Can you work these out from the model? Positions are in its coordinate system, mm. Face numbers are marked on the shaded views. A direction names the side the tool comes from. Round coordinates to 2 decimals unless told otherwise and drop trailing zeros. Order: outer loops, then holes, each group sorted by start corner. A loop starts at its lowest first (then second) coordinate and runs counter-clockwise, first axis right, second up. Notation, with made-up numbers: (-6, 37) -> (26, 37) arc R7 ccw to (26, 41) -> close; hole circle Ø5 at (13.5, -7). An arc over 180 degrees is marked (long way). Use a Markdown table: item, result. Add a question column.
Q1. If we section it at A-A on x = -2.15: List the corners of the cut face in (y, z) for me, plus the area to 3 significant figures.
Q2. For the marked faces 1 and 2, which set-ups out of +Z, -Z, +X, -X, +Y, -Y let a thin tool reach every point of the face, with its end or its side?
Q3. If we section it at B-B on x = 9.5: List the corners of the cut face in (y, z) for me.
Q4. I'm going to push flat-ended pins straight in: pin 1 Ø2 at (x, z) = (7.5, 3.5) entering from +Y; pin 2 Ø5 at (x, y) = (26, 4.5) entering from -Z; pin 3 Ø4 at (y, z) = (-2.5, 1) entering from +X; pin 4 Ø4 at (x, y) = (14, -3) entering from -Z. Where does each tip first touch, or does it pass through?
Q5. I need wall thicknesses on line 1 along X through (y, z) = (0, -3.9); line 2 along X through (y, z) = (0, -1.6); line 3 along X through (y, z) = (1.75, 4). Which ranges of each line are inside material? Lowest first, please. Write a range as [from, to].
Autodesk Inventor part; units mm, degrees
ref_plane "Work Plane1" through (16, 0, 0) normal (0, 0, -1) x (1, 0, 0)
ref_plane "YZ Plane" through (0, 0, 0) normal (1, 0, 0) x (0, 1, 0)
ref_plane "XZ Plane" through (0, 0, 0) normal (0, 1, 0) x (-1, 0, 0)
sketch "草图1" plane through (0, 0, 0) normal (0, 0, 1) x (1, 0, 0)
  line L0 (0, 4.45) -> (0, 3)
  line L1 (12, 3) -> (30, 3)
  line L2 (30, 3) -> (30, 0)
  line L3 (30, 0) -> (-0.1501, 0)
  line L4 (-6.1801, 0) -> (36.03, 0)
  line L5 (-0.1501, 0) -> (-0.1501, 4.45)
  line L6 (-0.1501, 4.45) -> (0, 4.45)
  line L7 (12, 3) -> (11.3866, 3)
  line L8 (11.3866, 3) -> (0, 3)
  line L9 (0, -0.89) -> (0, 5.34)
  line L10 (11.3866, 3) -> (11.3866, 0) construction
  line L11 (12, 3) -> (12, 0) construction
  dimension "d0" = 30
  dimension "d1" = 18
  dimension "d2" = 6
  dimension "d9" = 0.1501
  dimension "d10" = 8.9
  dimension "d13" = 0.6135
  dimension "d14" = 6
revolve "轴承体" add sketch "草图1" angle 360 about axis through (30, 0, 0) along (-1, 0, 0)
sketch "草图2" plane through (-0.1501, 0, 0) normal (-1, 0, 0) x (0, 0, 1)
  line L0 (0, 5.7735) -> (5, 2.8868)
  line L1 (5, 2.8868) -> (5, -2.8868)
  line L2 (5, -2.8868) -> (0, -5.7735)
  line L3 (0, -5.7735) -> (-5, -2.8868)
  line L4 (-5, -2.8868) -> (-5, 2.8868)
  line L5 (-5, 2.8868) -> (0, 5.7735)
  point P0 (0, 0)
  point P1 (0, 0)
  dimension "d11" = 10
extrude "头" add sketch "草图2" along normal blind 3.85
sketch "草图3" plane through (0, 0, 0) normal (0, 0, 1) x (1, 0, 0)
  line L0 (-4.0001, 5) -> (-4.0001, 5.7735)
  line L1 (-4.0001, 5.7735) -> (-3.5535, 5.7735)
  line L2 (-3.5535, 5.7735) -> (-4.0001, 5)
  line L3 (-4.7701, 0) -> (0.6199, 0)
  line L4 (-0.1501, 5.7735) -> (-4.0001, 5.7735)
  line L5 (-4.0001, 2.8868) -> (-4.0001, 5.7735)
  dimension "d5" = 30
  dimension "d25" = 10
revolve "倒角1" cut sketch "草图3" angle 360 about axis through (-10, 0, 0) along (1, 0, 0)
sketch "草图4" plane through (0, 0, 0) normal (0, 0, 1) x (1, 0, 0)
  circle A0 centre (-2.15, 0) radius 0.8
  line L0 (-3.54, 0) -> (0.59, 0)
  point P0 (0, 0)
  dimension "d18" = 1.6
  dimension "d19" = 2.15
extrude "孔" cut sketch "草图4" along normal through all both and the other way through all
pattern_circular "IDS_ARRAYHOLE" count 2 over 60 about axis through (-10, 0, 0) along (1, 0, 0) of "孔"
fillet "圆角1" radius 0.25 1 edges at (0, -3, 0)
thread "螺纹"
chamfer "倒角2" distance 0.6135 distance2 0.6136 1 edges at (30, -3, 0) measured on face at (30, -0.5525, 1.8157)
ref_plane "Work Plane1" through (16, 0, 0) normal (0, 0, -1) x (1, 0, 0)
equation "\"d0\" = NLG"
equation "\"d1\" = GEL"
equation "\"d2\" = GD"
equation "\"d10\" = SD2"
equation "\"d13\" = GAL"
equation "\"d14\" = BDM"
equation "\"d11\" = SW"
equation "\"d3\" = KOH - SD"
equation "\"d5\" = ANG1"
equation "\"d25\" = SW0"
equation "\"d18\" = BOR"
equation "\"d24\" = RR"
equation "\"d15\" = GEL"
equation "\"d6\" = -0.5 * SPD + 0.5 * GD"
equation "\"NLG\" = 30"
equation "\"GD\" = NND"
equation "\"BDM\" = NND"
equation "\"KOH\" = 4"
equation "\"GEL\" = 18"
equation "\"SW\" = 10"
equation "\"SW0\" = SW"
equation "\"SPD\" = NND - 1.2269 * PTC"
equation "\"SD2\" = SDH"
equation "\"SD\" = WFT"
equation "\"ANG1\" = 30deg"
equation "\"GAL\" = 0.61345 * PTC"
equation "\"GUL\" = 0.61345 * PTC"
equation "\"DIST\" = 2"
equation "\"BOR\" = 1.6"
equation "\"RR\" = 0.25"
equation "\"WFT\" = 0.15"
equation "\"FAWI\" = 45deg"
equation "\"PTC\" = 1"
equation "\"THREADDIA\" = 6"
equation "\"E0\" = 1.155 * SW"
equation "\"TOA\" = 30deg"
equation "\"NND\" = 6"
equation "\"GD1\" = THREADDIA - 1.2269 * PTC"
equation "\"SDH\" = 8.9"
properties part number "螺栓 GB 32.1 M6 x 30" material "钢，软"
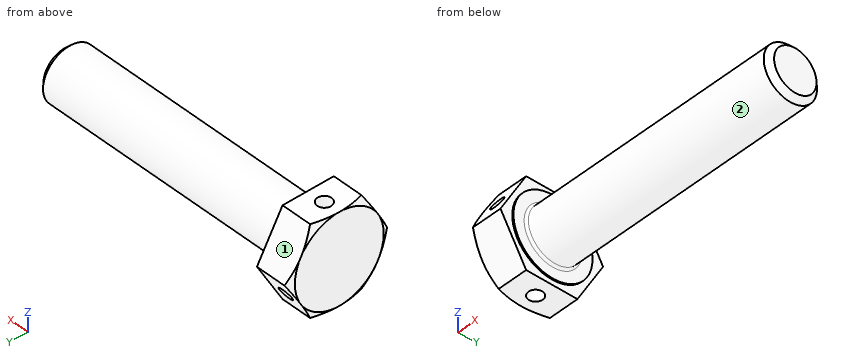
Answer below:
| question | item | result |
|---|---|---|
| 1 | outline | (-5.77, 0) -> (-2.89, -5) -> (-0.8, -5) -> (-0.8, -0.46) -> (-4.73, 1.81) -> close; (-3.93, 3.19) -> (-0.8, 1.39) -> (-0.8, 5) -> (-2.89, 5) -> close; (0.8, -5) -> (2.89, -5) -> (3.93, -3.19) -> (0.8, -1.39) -> close; (0.8, 0.46) -> (4.73, -1.81) -> (5.77, 0) -> (2.89, 5) -> (0.8, 5) -> close |
| 1 | area | 57.6 mm² |
| 2 | face 1 | +Z, +X, -X, +Y |
| 2 | face 2 | +X |
| 3 | outline | circle Ø6 at (0, 0) |
| 4 | pin 1 | y = 1.66 |
| 4 | pin 2 | z = -2.24 |
| 4 | pin 3 | x = 30 |
| 4 | pin 4 | z = -2.83 |
| 5 | line 1 | [-4, -2.95], [-1.35, 0] |
| 5 | line 2 | [-4, -2.95], [-1.35, 30] |
| 5 | line 3 | [-4, 0] |
